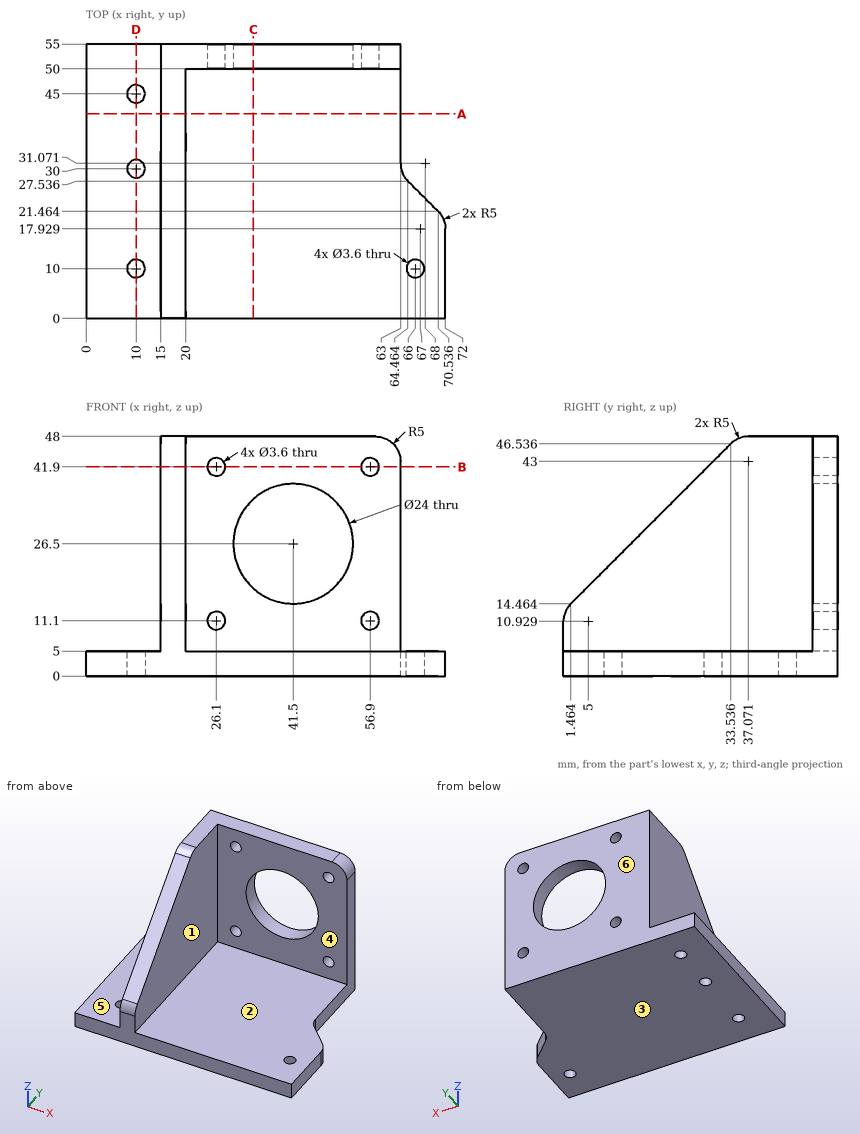
Input: dimensioned drawing with shaded views. Units: mm. Origin: part minimum x, y, z. A direction names the side the tool comes from. Give positions to 0.01 mm unless a question says otherwise; leave off trailing zeros. Write each loop counter-clockwise with the first axis right and the second up, starting at its lowest first coordinate (ties: lowest second). Pieces come first, ordered by that corner, then holes.
Q1. First-contact query: P1, Ø6, axis at y = 34, z = 31.5, coming from the -X side; P2, Ø1.5, axis at x = 27.5, y = 34, coming from the +Z side; P3, Ø19, axis at y = 47.5, z = 31, coming from the +X side. Flat tips, straight axial feed; report the tip coordinate or a pass-through.
Q2. Set-up query: the marked faces 4, 5 and 6. Return all of +Z, -Z, +X, -X, +Y, -Y with unobstructed straight access to the full face (end or side cutting, diameter ignored); none if empty.
Q3. Section D-D, the plane x = 10. Output: boundary loops of the cut face in (y, z), plus the area to 3 significant figures.
Q4. Section C-C, the plane x = 33.5. Output: boundary loops of the cut face in (y, z) (1 decimal).
Q5. Pull-direction query (Z, two-part tool) for the marked faces 1, 2 and 3; classes: pulls with the +Z half, pulls with the -Z half, needs draft (parallel to the pull), parting line crosses it, or undercut.
Q6. Section A-A, the plane y = 41. Output: boundary loops of the cut face in (x, z).
Q7. Material intervals for probe 1 along Y at (x, z) = (10, 3.3); probe 2 along Z at (x, y) = (6, 19); probe 3 along X at (y, z) = (37, 18.5), sorted ascending.
Q8. Section B-B, the plane z = 41.9. Output: boundary loops of the cut face in (x, y).
Filled in:
1. P1: stops at x = 15
1. P2: stops at z = 5
1. P3: stops at x = 63
2. face 4: +Z, +X, -Y
2. face 5: +Z, -X, +Y, -Y
2. face 6: +Z, -Z, +X, -X, +Y
3. outline: (0, 0) - (8.2, 0) - (8.2, 5) - (0, 5) - close; (11.8, 0) - (28.2, 0) - (28.2, 5) - (11.8, 5) - close; (31.8, 0) - (43.2, 0) - (43.2, 5) - (31.8, 5) - close; (46.8, 0) - (55, 0) - (55, 5) - (46.8, 5) - close
3. area: 221 mm2
4. outline: (0, 0) - (55, 0) - (55, 17.6) - (50, 17.6) - (50, 5) - (0, 5) - close; (50, 35.4) - (55, 35.4) - (55, 48) - (50, 48) - close
5. face 1: needs draft
5. face 2: pulls with the +Z half
5. face 3: pulls with the -Z half
6. outline: (0, 0) - (63, 0) - (63, 5) - (20, 5) - (20, 48) - (15, 48) - (15, 5) - (0, 5) - close
7. probe 1: y = 0 to 8.2, 11.8 to 28.2, 31.8 to 43.2, 46.8 to 55
7. probe 2: z = 0 to 5
7. probe 3: x = 15 to 20
8. outline: (15, 28.9) - (20, 28.9) - (20, 50) - (24.3, 50) - (24.3, 55) - (15, 55) - close; (27.9, 50) - (55.1, 50) - (55.1, 55) - (27.9, 55) - close; (58.7, 50) - (63, 50) - (63, 55) - (58.7, 55) - close
